```python
from build123d import *

# Parameters (mm, degrees)
BOSS_EXTRUDE1_DEPTH     = 33.8
CUT_EXTRUDE1_DEPTH      = 23
CUT_EXTRUDE1_DEPTH_BACK = 23


with BuildPart() as part:
    # Sketch1 → Boss-Extrude1 (new body)
    with BuildSketch(Plane(origin=(0, 1.3, 0), x_dir=(1, 0, 0), z_dir=(0, 1, 0))):
        with BuildLine():
            Line((0, -22.541858429), (0, -53.65))
            Line((0, -53.65), (18, -53.65))
            Line((18, -53.65), (18, -22.654162541))
            ThreePointArc((18, -22.654162541), (17.938748215, -22.414370958), (17.769999986, -22.233330024))
            ThreePointArc((17.769999986, -22.233330024), (16.858228534, -20.731235829), (17.483912522, -19.089245057))
            Line((17.483912522, -19.089245057), (18.57947873, -18.064679449))
            ThreePointArc((18.57947873, -18.064679449), (19.138283161, -16.544955286), (18.250000071, -15.191154314))
            ThreePointArc((18.250000071, -15.191154314), (18.066987319, -15.008141607), (18, -14.758141571))
            Line((18, -14.758141571), (18, 53.65))
            Line((18, 53.65), (0, 53.65))
            Line((0, 53.65), (0, -14.645837459))
            ThreePointArc((0, -14.645837459), (0.061251781, -14.885629035), (0.23, -15.066669967))
            ThreePointArc((0.23, -15.066669967), (1.141771466, -16.568764162), (0.516087478, -18.210754943))
            Line((0.516087478, -18.210754943), (-0.57947873, -19.235320551))
            ThreePointArc((-0.57947873, -19.235320551), (-1.138283159, -20.755044733), (-0.250000037, -22.108845706))
            ThreePointArc((-0.250000037, -22.108845706), (-0.066987309, -22.29185841), (0, -22.541858429))
        make_face()
    extrude(amount=BOSS_EXTRUDE1_DEPTH)

    # Sketch2 → Cut-Extrude1 (cut, two sides)
    with BuildSketch(Plane(origin=(0, 0, 0), x_dir=(0, 0, -1), z_dir=(1, 0, 0))) as cut_extrude1_sk:
        Polygon((-26, 2.9), (-26, -8.174443219), (14, -7.963716906), (14, 2.543524479), (16.45, 3.2), (16.45, 4.4), (-19.05, 4.4), (-19.05, 2.9), align=None)
    extrude(amount=CUT_EXTRUDE1_DEPTH, mode=Mode.SUBTRACT)
    extrude(cut_extrude1_sk.sketch, amount=-CUT_EXTRUDE1_DEPTH_BACK, mode=Mode.SUBTRACT)

    # Sketch3 → Cut-Revolve1 (revolve, cut)
    with BuildSketch(Plane(origin=(9, 0, 0), x_dir=(0, 0, -1), z_dir=(1, 0, 0))):
        Polygon((-53.65, 9.8), (-53.65, 16.3785), (-52.794, 15.5225), (-40.65, 15.5225), (-40.65, 9.8), align=None)
    revolve(axis=Axis((9, 9.8, 40.65), (0, 0, 1)), mode=Mode.SUBTRACT)

    # Sketch4 → Cut-Revolve2 (revolve, cut)
    with BuildSketch(Plane(origin=(12, 0, 0), x_dir=(0, 0, -1), z_dir=(1, 0, 0))):
        Polygon((-53.65, 23.86), (-53.65, 27.36), (-53.1085, 26.8185), (-46.65, 26.8185), (-46.65, 23.86), align=None)
    revolve(axis=Axis((12, 23.86, 46.65), (0, 0, 1)), mode=Mode.SUBTRACT)

    # Sketch5 → Cut-Revolve3 (revolve, cut)
    with BuildSketch(Plane(origin=(3.1, 0, 0), x_dir=(0, 0, -1), z_dir=(1, 0, 0))):
        Polygon((-38.05, 35.1), (-36.55, 35.1), (-36.8205, 34.8295), (-36.8205, 30.1), (-38.05, 30.1), align=None)
    revolve(axis=Axis((3.1, 30.1, 38.05), (0, 1, 0)), mode=Mode.SUBTRACT)

    # Sketch6 → Cut-Revolve4 (revolve, cut)
    with BuildSketch(Plane(origin=(3.1, 0, 0), x_dir=(0, 0, -1), z_dir=(1, 0, 0))):
        Polygon((0.75, 35.1), (2.25, 35.1), (1.9795, 34.8295), (1.9795, 30.1), (0.75, 30.1), align=None)
    revolve(axis=Axis((3.1, 30.1, -0.75), (0, 1, 0)), mode=Mode.SUBTRACT)

    # Sketch7 → Cut-Revolve5 (revolve, cut)
    with BuildSketch(Plane(origin=(3.1, 0, 0), x_dir=(0, 0, -1), z_dir=(1, 0, 0))):
        Polygon((50.75, 35.1), (52.25, 35.1), (51.9795, 34.8295), (51.9795, 30.1), (50.75, 30.1), align=None)
    revolve(axis=Axis((3.1, 30.1, -50.75), (0, 1, 0)), mode=Mode.SUBTRACT)

    # Sketch8 → Cut-Revolve6 (revolve, cut)
    with BuildSketch(Plane(origin=(14.9, 0, 0), x_dir=(0, 0, -1), z_dir=(1, 0, 0))):
        Polygon((-38.05, 35.1), (-36.55, 35.1), (-36.8205, 34.8295), (-36.8205, 30.1), (-38.05, 30.1), align=None)
    revolve(axis=Axis((14.9, 30.1, 38.05), (0, 1, 0)), mode=Mode.SUBTRACT)

    # Sketch9 → Cut-Revolve7 (revolve, cut)
    with BuildSketch(Plane(origin=(14.9, 0, 0), x_dir=(0, 0, -1), z_dir=(1, 0, 0))):
        Polygon((0.75, 35.1), (2.25, 35.1), (1.9795, 34.8295), (1.9795, 30.1), (0.75, 30.1), align=None)
    revolve(axis=Axis((14.9, 30.1, -0.75), (0, 1, 0)), mode=Mode.SUBTRACT)

    # Sketch10 → Cut-Revolve8 (revolve, cut)
    with BuildSketch(Plane(origin=(14.9, 0, 0), x_dir=(0, 0, -1), z_dir=(1, 0, 0))):
        Polygon((50.75, 35.1), (52.25, 35.1), (51.9795, 34.8295), (51.9795, 30.1), (50.75, 30.1), align=None)
    revolve(axis=Axis((14.9, 30.1, -50.75), (0, 1, 0)), mode=Mode.SUBTRACT)

    # Sketch11 → Cut-Revolve9 (revolve, cut)
    with BuildSketch(Plane(origin=(0, 13, 0), x_dir=(1, 0, 0), z_dir=(0, 1, 0))):
        Polygon((12.75, 53.65), (14.665, 53.65), (14.165, 53.15), (14.165, 44.65), (12.75, 43.833049369), align=None)
    revolve(axis=Axis((12.75, 13, -43.833049369), (0, 0, -1)), mode=Mode.SUBTRACT)

    # Sketch12 → Cut-Revolve10 (revolve, cut)
    with BuildSketch(Plane(origin=(0, 13, 0), x_dir=(1, 0, 0), z_dir=(0, 1, 0))):
        Polygon((5.25, 53.65), (7.165, 53.65), (6.665, 53.15), (6.665, 44.65), (5.25, 43.833049369), align=None)
    revolve(axis=Axis((5.25, 13, -43.833049369), (0, 0, -1)), mode=Mode.SUBTRACT)


solid = part.part
```
Source: CAD feature listing. Evaluate the final solid. Frame: model axes, mm. A direction names the side the tool comes from. Round coordinates to 2 decimals unless told otherwise and drop trailing zeros. Loops run counter-clockwise (first coordinate to the right, second up) from the corner with the lowest first, then second, coordinate; pieces in that order, holes last. Notation, with made-up numbers: M 80,85 L 123,85 A19 ccw 123,98 Z; hole C 48.5,37.25 d3. An arc over 180 degrees is marked long. Use a Markdown table: item, result. Add a question column.
1. Ray query, line 1 along Z through (x, y) = (14.9, 33.6); line 2 along X through (y, z) = (31.4, 38.05); line 3 along X through (y, z) = (13, -46.75) (3 decimals). Return the intervals inside material, ascending. Write a range as [from, to].
2. Cut plane C-C, the plane z = 38.05. Output: boundary loops of the cut face in (x, y), and give its area (3 significant figures).
3. Cut plane D-D, the plane y = 23.86. Output: boundary loops of the cut face in (x, z).
4. Cut plane B-B, the plane y = 9.8. Output: boundary loops of the cut face in (x, z), and give its area (3 significant figures).
5. Contact query for flat-ended pins moving along their axis: pin 1 (2 mm diameter, centred on x = 14.9, z = -50.75, fed in from +Y); pin 2 (3 mm diameter, centred on x = 2, z = 20, fed in from -Y); pin 3 (1.2 mm diameter, centred on x = 2.5, z = 37.5, fed in from +Y). Output: stop coordinate, or through.
6. Pull-direction query (X, two-part tool) for faces 5 (the flat face through (18, 18, 38)), 6 (the flat face through (11, 35.1, -1)), 7 (the cylindrical face through (5.066, 11.597, -48.84)); classes: +X half, -X half, draft (parallel to the pull), parting line (faces both ways), or undercut.
7. Cut plane A-A, the plane y = 32.5. Output: boundary loops of the cut face in (x, z), and give its area (3 significant figures).
8. Set-up query: faces 1 (the flat face through (0, 18, -20)), 2 (the cylindrical face through (3.326, 9.055, 46.637)), 3 (the cylindrical face through (13.5, 11.8, -48.8)), 4 (the cylindrical face through (2.731, 32.432, -1.923)). Return all of +Z, -Z, +X, -X, +Y, -Y with unobstructed straight access to the full face (end or side cutting, diameter ignored); none if empty.
Solution:
| question | item | result |
|---|---|---|
| 1 | line 1 | z = [-53.65, -51.98], [-49.52, -1.98], [0.48, 36.82], [39.28, 53.65] |
| 1 | line 2 | x = [0, 1.87], [4.33, 13.67], [16.13, 18] |
| 1 | line 3 | x = [0, 3.835], [6.665, 11.335], [14.165, 18] |
| 2 | outline | M 0,1.3 L 18,1.3 L 18,35.1 L 16.4,35.1 L 16.13,34.83 L 16.13,30.1 L 13.67,30.1 L 13.67,34.83 L 13.4,35.1 L 4.6,35.1 L 4.33,34.83 L 4.33,30.1 L 1.87,30.1 L 1.87,34.83 L 1.6,35.1 L 0,35.1 Z |
| 2 | area | 584 mm2 |
| 3 | outline | M -0.58,19.24 L 0.52,18.21 A2 cw 0.23,15.07 A0.5 ccw 0,14.65 L 0,-53.65 L 18,-53.65 L 18,14.76 A0.5 cw 18.25,15.19 A1.8 ccw 18.58,18.06 L 17.48,19.09 A2 cw 17.77,22.23 A0.5 ccw 18,22.65 L 18,53.65 L 15.5,53.65 L 14.96,53.11 L 14.96,46.65 L 9.04,46.65 L 9.04,53.11 L 8.5,53.65 L 0,53.65 L 0,22.54 A0.5 cw -0.25,22.11 A1.8 ccw Z |
| 4 | outline | M -0.58,19.24 L 0.52,18.21 A2 cw 0.23,15.07 A0.5 ccw 0,14.65 L 0,-53.65 L 18,-53.65 L 18,14.76 A0.5 cw 18.25,15.19 A1.8 ccw 18.58,18.06 L 17.48,19.09 A2 cw 17.77,22.23 A0.5 ccw 18,22.65 L 18,53.65 L 15.58,53.65 L 14.72,52.79 L 14.72,40.65 L 3.28,40.65 L 3.28,52.79 L 2.42,53.65 L 0,53.65 L 0,22.54 A0.5 cw -0.25,22.11 A1.8 ccw Z |
| 4 | area | 1,780 mm2 |
| 5 | pin 1 | stops at y = 30.1 |
| 5 | pin 2 | stops at y = 2.9 |
| 5 | pin 3 | stops at y = 35.01 |
| 6 | face 5 | +X half |
| 6 | face 6 | draft |
| 6 | face 7 | undercut |
| 7 | outline | M -0.58,19.24 L 0.52,18.21 A2 cw 0.23,15.07 A0.5 ccw 0,14.65 L 0,-53.65 L 18,-53.65 L 18,14.76 A0.5 cw 18.25,15.19 A1.8 ccw 18.58,18.06 L 17.48,19.09 A2 cw 17.77,22.23 A0.5 ccw 18,22.65 L 18,53.65 L 0,53.65 L 0,22.54 A0.5 cw -0.25,22.11 A1.8 ccw Z; hole C 3.1,-50.75 d2.46; hole C 3.1,-0.75 d2.46; hole C 3.1,38.05 d2.46; hole C 14.9,-50.75 d2.46; hole C 14.9,-0.75 d2.46; hole C 14.9,38.05 d2.46 |
| 7 | area | 1,900 mm2 |
| 8 | face 1 | -Z, -X, +Y, -Y |
| 8 | face 2 | +Z |
| 8 | face 3 | -Z |
| 8 | face 4 | +Y |
